from build123d import *

# Parameters (mm, degrees)
SKETCH_1_W          = 3
SKETCH_1_H          = 2.75
SKETCH_2_R          = 1.5
EXTRUDE_1_DEPTH     = 16
CUT_EXTRUDE_1_DEPTH = 1.3
CHAMFER_1_SIZE      = 0.3


with BuildPart() as part:
    # 草图1 → 旋转1 (revolve)
    with BuildSketch(Plane(origin=(0, 0, 0), x_dir=(-1, 0, 0), z_dir=(0, 0, -1))):
        with Locations((-1.5, 1.375)):
            Rectangle(SKETCH_1_W, SKETCH_1_H)
    revolve(axis=Axis((3, 0, 0), (-1, 0, 0)))

    # 草图2 → 凸台-拉伸1 (add)
    with BuildSketch(Plane(origin=(3, 0, 0), x_dir=(0, 0, -1), z_dir=(1, 0, 0))):
        Circle(SKETCH_2_R)
    extrude(amount=EXTRUDE_1_DEPTH)

    # 草图3 → 切除-拉伸1 (cut)
    with BuildSketch(Plane.ZY):
        Polygon((1.28, 0.739008345), (0, 1.478016689), (-1.28, 0.739008345), (-1.28, -0.739008345), (0, -1.478016689), (1.28, -0.739008345), align=None)
    extrude(amount=-CUT_EXTRUDE_1_DEPTH, mode=Mode.SUBTRACT)

    # 草图4 → 切除-旋转1 (revolve, cut)
    with BuildSketch(Plane.XY):
        Polygon((1.3, 1.28), (1.3, 0), (2.039008345, 0), align=None)
    revolve(axis=Axis((1.3, 0, 0), (1, 0, 0)), mode=Mode.SUBTRACT)

    # 倒角1
    chamfer_1_edges = [part.edges().sort_by_distance(p)[0] for p in [
        (19, 0, 1.5),
        (0, -2.75, 0),
    ]]
    chamfer(chamfer_1_edges, length=CHAMFER_1_SIZE)


solid = part.part
Geometry: final body of the model. Coordinates: model frame, mm. A direction names the side the tool comes from. Give positions to 0.01 mm unless a question says otherwise; leave off trailing zeros. Order: outer loops, then holes, each group sorted by start corner. A loop starts at its lowest first (then second) coordinate and runs counter-clockwise, first axis right, second up. Notation, with made-up numbers: (87.25, 70) -> (106.25, 70) arc R23 cw to (106.25, 98) -> close; hole circle Ø5 at (-20, 78.25). An arc over 180 degrees is marked (long way). Put each result on its own line as item: value.
Q1. Reachability of faces 1 (the face through (0.641, -1.103, -0.649)), 2 (the face through (10.74, 0.07, 1.5)), 3 (the face through (19, 0, 0)) from +Z, -Z, +X, -X, +Y, -Y: full face, straight path, thin tool, end or side. Return the list, or none.
Here are the results:
face 1: -X
face 2: +X
face 3: +Z, -Z, +X, +Y, -Y
Q2. Section A-A, the plane x = 6. Return loops of the section in (y, z), then the cut area to 3 significant figures.
Here are the results:
outline: circle Ø3 at (0, 0)
area: 7.07 mm^2
Q3. Pin query (flat end, axial travel): pin 1 (0.5 mm diameter, centred on y = -0.5, z = -1, fed in from -X); pin 2 (3 mm diameter, centred on x = 7.5, z = 0.5, fed in from -Y); pin 3 (2 mm diameter, centred on x = 15.5, z = -2, fed in from -Y). Return the tip coordinate at first contact, or that it passes through.
Here are the results:
pin 1: stops at x = 1.3
pin 2: stops at y = -1.5
pin 3: stops at y = -1.12
Q4. Draft query along Y for faces 4 (the face through (1.631, -0.596, 2.685)), 5 (the face through (0.641, 1.114, -0.631)), 6 (the face through (3, -1.2, 1.2)). Return one class per face: released by +Y, released by -Y, zero draft, split by the parting line, or undercut.
Here are the results:
face 4: split by the parting line
face 5: undercut
face 6: zero draft
Q5. Section B-B, the plane x = 1.5. Return loops of the section in (y, z).
Here are the results:
outline: circle Ø5.5 at (0, 0); hole circle Ø1.87 at (0, 0)
Q6. Material intervals for L1, parallel to Y at x = 18, z = 0; L2, parallel to X at y = -1.75, z = -0.8; L3, parallel to Y at x = 17.5, z = 1.3, sorted ascending.
Here are the results:
L1: y = -1.5 to 1.5
L2: x = 0 to 3
L3: y = -0.75 to 0.75
